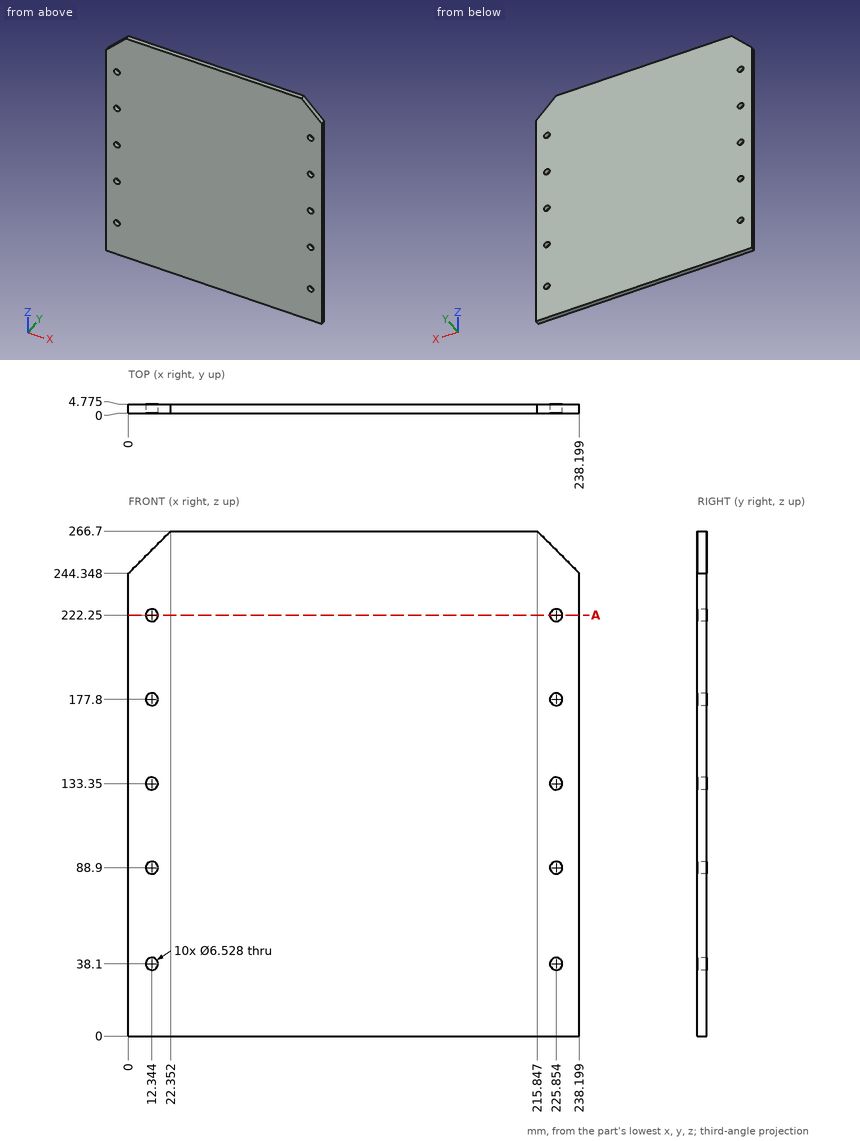
Geometry: see drawing. Coordinates: mm, zero at the bounding-box minimum. Round coordinates to 2 decimals unless told otherwise and drop trailing zeros. Order: outer loops, then holes, each group sorted by start corner. A loop starts at its lowest first (then second) coordinate and runs counter-clockwise, first axis right, second up. Notation, with made-up numbers: (9, -14.5) -> (16, -14.5) arc R33 cw to (16, 15.5) -> close; hole circle Ø9 at (9.25, 75.25). An arc over 180 degrees is marked (long way). Use CSV: the item, a comma, the result in double quotes.
(1) First-contact query: pin 1 Ø6 at (x, z) = (12.34, 38.1) entering from +Y; pin 2 Ø2 at (x, y) = (127.5, 2.5) entering from -Z. Flat tips, straight axial feed; report the tip coordinate or a pass-through.
Report:
pin 1,"through"
pin 2,"z = 0"
(2) Section A-A on z = 222.25. Return the cut outline in (x, y) (1 decimal), and give its area (4 significant figures).
Report:
outline,"(0, 0) -> (9.1, 0) -> (9.1, 4.8) -> (0, 4.8) -> close; (15.6, 0) -> (222.6, 0) -> (222.6, 4.8) -> (15.6, 4.8) -> close; (229.1, 0) -> (238.2, 0) -> (238.2, 4.8) -> (229.1, 4.8) -> close"
area,"1,075 mm^2"
(3) Ray query, L1, parallel to X at y = 2.2, z = 38.1; L2, parallel to X at y = 3.2, z = 39; L3, parallel to Z at x = 17.5, y = 4.4. Return the intervals inside material, ascending.
Report:
L1,"0 to 9.08, 15.61 to 222.59, 229.12 to 238.2"
L2,"0 to 9.21, 15.48 to 222.72, 228.99 to 238.2"
L3,"0 to 261.85"
